```python
from build123d import *

# Parameters (mm, degrees)
SKETCH1_W           = 50.8
SKETCH1_H           = 50.8
BOSS_EXTRUDE1_DEPTH = 50.8
SKETCH2_R           = 6.35
BOSS_EXTRUDE2_DEPTH = 76.2


with BuildPart() as part:
    # Sketch1 → Boss-Extrude1 (new body)
    with BuildSketch(Plane(origin=(0, 0, 0), x_dir=(1, 0, 0), z_dir=(0, 1, 0))):
        with Locations((0, 0.779824561)):
            Rectangle(SKETCH1_W, SKETCH1_H)
    extrude(amount=BOSS_EXTRUDE1_DEPTH)

    # Sketch2 → Boss-Extrude2 (add)
    with BuildSketch(Plane(origin=(0, 50.8, 0), x_dir=(1, 0, 0), z_dir=(0, 1, 0))):
        Circle(SKETCH2_R)
    extrude(amount=BOSS_EXTRUDE2_DEPTH)


solid = part.part
```
Could you check a few things on this model? Use its own coordinates, in mm. A direction names the side the tool comes from. Round coordinates to 2 decimals unless told otherwise and drop trailing zeros. Write each loop counter-clockwise with the first axis right and the second up, starting at its lowest first coordinate (ties: lowest second). Pieces come first, ordered by that corner, then holes.
(1) Suppose I cut it at D-D on z = 18.5. Write out the boundary of the cut face in (x, y).
Findings below:
outline: (-25.4, 0) - (25.4, 0) - (25.4, 50.8) - (-25.4, 50.8) - close
(2) Suppose I cut it at B-B on x = 0. Write out the boundary of the cut face in (y, z).
Findings below:
outline: (0, -26.18) - (50.8, -26.18) - (50.8, -6.35) - (127, -6.35) - (127, 6.35) - (50.8, 6.35) - (50.8, 24.62) - (0, 24.62) - close
(3) Suppose I cut it at C-C on y = 112.5. Write out the boundary of the cut face in (x, z), and give its area (3 significant figures).
Findings below:
outline: circle Ø12.7 at (0, 0)
area: 127 mm2
(4) Suppose I cut it at A-A on z = 0. Write out the boundary of the cut face in (x, y).
Findings below:
outline: (-25.4, 0) - (25.4, 0) - (25.4, 50.8) - (6.35, 50.8) - (6.35, 127) - (-6.35, 127) - (-6.35, 50.8) - (-25.4, 50.8) - close
(5) For pin 1 (6 mm diameter, centred on x = 4.5, z = 18, fed in from +Y), with a flat end and sliding along its axis, tell me the tip position at first contact or that it passes through.
Findings below:
pin 1: stops at y = 50.8
(6) Which directions (+Z, -Z, +X, -X, +Y, -Y) give clear straight access to the entire face, cutting with the end or side of a thin tool? Please do faces 1 (the face through (-1.38, 88.37, 6.2)), 2 (the face through (0, 0, -1)).
Findings below:
face 1: +Y
face 2: +Z, -Z, +X, -X, -Y
(7) If I drill on probe 1 along Y at (x, z) = (-9, 7); probe 2 along X at (y, z) = (72, -0.5); probe 3 along X at (y, z) = (116, 4.5), over which ranges is the centre line in solid material (lowest first)?
Findings below:
probe 1: y = 0 to 50.8
probe 2: x = -6.33 to 6.33
probe 3: x = -4.48 to 4.48
